```python
from build123d import *

# Parameters (mm, degrees)
SKETCH_1_W          = 20
SKETCH_1_H          = 40
SKETCH_1_W_2        = 18
SKETCH_1_H_2        = 38
EXTRUDE_1_DEPTH     = 240
SKETCH_2_R          = 1.6
CUT_EXTRUDE_1_DEPTH = 280
SKETCH_3_R          = 1.6
CUT_EXTRUDE_2_DEPTH = 280


with BuildPart() as part:
    # 草图1 → 凸台-拉伸1 (new body)
    with BuildSketch(Plane.XY):
        with Locations((10, 20)):
            Rectangle(SKETCH_1_W, SKETCH_1_H)
        with Locations((10, 20)):
            Rectangle(SKETCH_1_W_2, SKETCH_1_H_2, mode=Mode.SUBTRACT)
    extrude(amount=EXTRUDE_1_DEPTH)

    # 草图2 → 切除-拉伸1 (cut)
    with BuildSketch(Plane(origin=(0, 40, 0), x_dir=(1, 0, 0), z_dir=(0, 1, 0))):
        with Locations(Location((6, -221, 0), (0, 0, 270))):
            Circle(SKETCH_2_R)
        with Locations(Location((6, -233, 0), (0, 0, 270))):
            Circle(SKETCH_2_R)
        with Locations((34, -221)):
            Circle(SKETCH_2_R)
        with Locations((34, -233)):
            Circle(SKETCH_2_R)
        with Locations(Location((4, -191, 0), (0, 0, 270))):
            Circle(SKETCH_2_R)
        with Locations(Location((4, -181, 0), (0, 0, 270))):
            Circle(SKETCH_2_R)
        with Locations(Location((16, -167, 0), (0, 0, 270))):
            Circle(SKETCH_2_R)
        with Locations(Location((16, -157, 0), (0, 0, 270))):
            Circle(SKETCH_2_R)
        with Locations(Location((4, -167, 0), (0, 0, 270))):
            Circle(SKETCH_2_R)
        with Locations(Location((4, -157, 0), (0, 0, 270))):
            Circle(SKETCH_2_R)
        with Locations(Location((16, -191, 0), (0, 0, 270))):
            Circle(SKETCH_2_R)
        with Locations(Location((16, -181, 0), (0, 0, 270))):
            Circle(SKETCH_2_R)
    extrude(amount=-CUT_EXTRUDE_1_DEPTH, mode=Mode.SUBTRACT)

    # 草图3 → 切除-拉伸2 (cut)
    with BuildSketch(Plane.ZY):
        with Locations((10, 8)):
            Circle(SKETCH_3_R)
        with Locations((34, 8)):
            Circle(SKETCH_3_R)
        with Locations((10, 32)):
            Circle(SKETCH_3_R)
        with Locations((34, 32)):
            Circle(SKETCH_3_R)
        with Locations((22, 32)):
            Circle(SKETCH_3_R)
        with Locations((22, 8)):
            Circle(SKETCH_3_R)
        with Locations((84, 24)):
            Circle(SKETCH_3_R)
        with Locations((94, 24)):
            Circle(SKETCH_3_R)
        with Locations((108, 36)):
            Circle(SKETCH_3_R)
        with Locations((118, 36)):
            Circle(SKETCH_3_R)
        with Locations((108, 24)):
            Circle(SKETCH_3_R)
        with Locations((118, 24)):
            Circle(SKETCH_3_R)
        with Locations((84, 36)):
            Circle(SKETCH_3_R)
        with Locations((94, 36)):
            Circle(SKETCH_3_R)
    extrude(amount=-CUT_EXTRUDE_2_DEPTH, mode=Mode.SUBTRACT)


solid = part.part
```
Build history of the part. All positions in model axes, mm. A direction names the side the tool comes from. Round coordinates to 2 decimals unless told otherwise and drop trailing zeros. Order: outer loops, then holes, each group sorted by start corner. A loop starts at its lowest first (then second) coordinate and runs counter-clockwise, first axis right, second up. Notation, with made-up numbers: (43, 86.25) -> (57, 86.25) arc R23 cw to (57, 110.25) -> close; hole circle Ø2 at (5, 0). An arc over 180 degrees is marked (long way). Answer in a Markdown table with one row per item.
1) Pin check, flat tip, straight feed: P1, Ø1.9, axis at y = 32, z = 34, coming from the +X side. Stop position of the tip, or through.
Values:
| item | result |
|---|---|
| P1 | through |
2) Which spindle directions (+Z, -Z, +X, -X, +Y, -Y) get a long thin tool onto all of the face, cutting with end or side? Do faces 5 (the flat face through (19, 20, 118)), 6 (the flat face through (0.3, 20.1, 240)). Say none if no direction does.
Values:
| item | result |
|---|---|
| face 5 | +Z, -Z |
| face 6 | +Z, +X, -X, +Y, -Y |
3) Mould opens along Y. For faces 1 (the flat face through (10, 0, 118)), 2 (the flat face through (10, 40, 118)), 3 (the flat face through (0, 20, 118)), 4 (the flat face through (1, 20, 118)) say: released by +Y, released by -Y, zero draft, split by the parting line, or undercut.
Values:
| item | result |
|---|---|
| face 1 | released by -Y |
| face 2 | released by +Y |
| face 3 | zero draft |
| face 4 | undercut |
4) Wall check: L1, parallel to Y at x = 19.7, z = 84; L2, parallel to Y at x = 0.8, z = 34; L3, parallel to Y at x = 16.5, z = 69. Give the ranges that are in metal, low to high.
Values:
| item | result |
|---|---|
| L1 | 0 to 22.4, 25.6 to 34.4, 37.6 to 40 |
| L2 | 0 to 6.4, 9.6 to 30.4, 33.6 to 40 |
| L3 | 0 to 1, 39 to 40 |
5) Band-saw the part on A-A on y = 14.5. Give the cut face in (x, z).
Values:
| item | result |
|---|---|
| outline | (0, 0) -> (1, 0) -> (1, 240) -> (0, 240) -> close; (19, 0) -> (20, 0) -> (20, 240) -> (19, 240) -> close |
6) Band-saw the part on B-B on z = 100.5. Give the cut face in (x, y), and give its area (3 significant figures).
Values:
| item | result |
|---|---|
| outline | (0, 0) -> (20, 0) -> (20, 40) -> (0, 40) -> close; hole (1, 1) -> (19, 1) -> (19, 39) -> (1, 39) -> close |
| area | 116 mm2 |
